Source: three-view drawing plus pictorial views. Frame: mm from the lowest corner of the part. A direction names the side the tool comes from. Give positions to 0.01 mm unless a question says otherwise; leave off trailing zeros. Loops run counter-clockwise (first coordinate to the right, second up) from the corner with the lowest first, then second, coordinate; pieces in that order, holes last.
1. Access query for the marked faces 4, 5 and 6. Directions: +Z, -Z, +X, -X, +Y, -Y. A direction counts if a zero-diameter tool reaches every point of the face in a straight line with its end or side. Return the directions, or none.
2. Section A-A, the plane y = 12.3. Output: boundary loops of the cut face in (x, z) (3 decimals), then the cut area to 3 significant figures.
3. Section D-D, the plane z = 6.5. Output: boundary loops of the cut face in (x, y).
4. Section C-C, the plane x = 12. Output: boundary loops of the cut face in (y, z), then the cut area to 3 significant figures.
5. Draft query along X for the marked faces 1, 2 and 3. Return one class per face: +X half, -X half, draft (parallel to the pull), parting line (faces both ways), or undercut.
6. First-contact query: P1, Ø5, axis at x = 14.5, z = 9.5, coming from the +Y side; P2, Ø12.5, axis at y = 10, z = 14.5, coming from the +X side. Flat tips, straight axial feed; report the tip coordinate or a pass-through.
7. Section B-B, the plane z = 15.7. Output: boundary loops of the cut face in (x, y) (3 decimals).
8. Material intervals for line 1 along X through (y, z) = (7, 11.5); line 2 along Y through (x, z) = (30.75, 15.7) (3 decimals), sorted ascending.
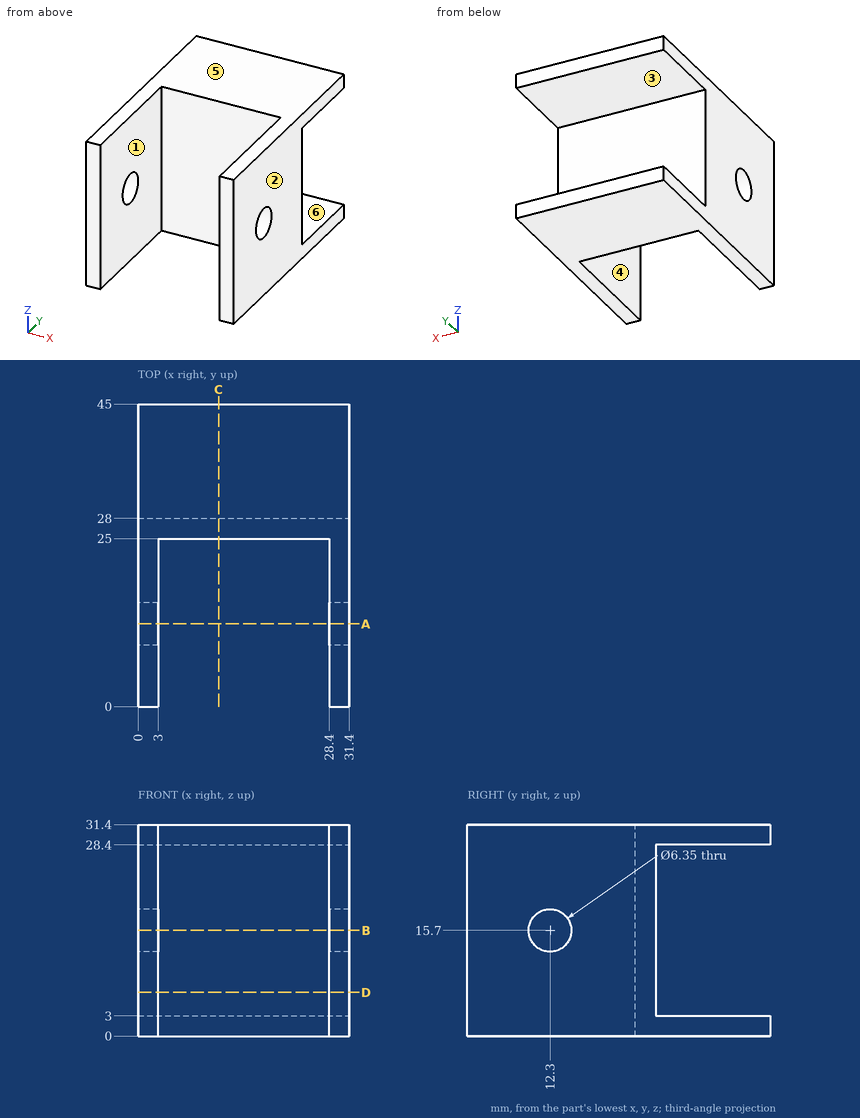
Answers below:
1. face 4: +Z, -Z, -Y
1. face 5: +Z, +X, -X, +Y, -Y
1. face 6: +X, -X, +Y
2. outline: (0, 0) - (3, 0) - (3, 12.525) - (0, 12.525) - close; (0, 18.875) - (3, 18.875) - (3, 31.4) - (0, 31.4) - close; (28.4, 0) - (31.4, 0) - (31.4, 12.525) - (28.4, 12.525) - close; (28.4, 18.875) - (31.4, 18.875) - (31.4, 31.4) - (28.4, 31.4) - close
2. area: 150 mm2
3. outline: (0, 0) - (3, 0) - (3, 25) - (28.4, 25) - (28.4, 0) - (31.4, 0) - (31.4, 28) - (0, 28) - close
4. outline: (25, 0) - (45, 0) - (45, 3) - (28, 3) - (28, 28.4) - (45, 28.4) - (45, 31.4) - (25, 31.4) - close
4. area: 196 mm2
5. face 1: undercut
5. face 2: +X half
5. face 3: draft
6. P1: stops at y = 28
6. P2: stops at x = 31.4
7. outline: (0, 0) - (3, 0) - (3, 9.125) - (0, 9.125) - close; (0, 15.475) - (3, 15.475) - (3, 25) - (28.4, 25) - (28.4, 15.475) - (31.4, 15.475) - (31.4, 28) - (0, 28) - close; (28.4, 0) - (31.4, 0) - (31.4, 9.125) - (28.4, 9.125) - close
8. line 1: x = 0 to 3, 28.4 to 31.4
8. line 2: y = 0 to 9.125, 15.475 to 28
